The drawing under review shows one solid part. Ordinate dimensions are in mm from its lowest x, y, z. A direction names the side the tool comes from. Coordinates: 2 decimals unless noted, no trailing zeros. Loops run counter-clockwise (first coordinate to the right, second up) from the corner with the lowest first, then second, coordinate; pieces in that order, holes last. Notation, with made-up numbers: (24, -38) - (28, -38) arc R23 ccw to (28, -10) - close; hole circle Ø10 at (55, 48). An arc over 180 degrees is marked (long way). Use one line per item in the form item = value. Start each with the question number.
1. Machinability: for the marked faces 1 and 2, which of the approach directions +Z, -Z, +X, -X, +Y, -Y give a long, thin tool a straight path to every point of the face, cutting with its end or side? Answer none if there is none.
2. Add section C-C on z = 15. Give the boundary of the cut face in (x, y).
3. Add section B-B on x = 21. Give the boundary of the cut face in (y, z), and give its area (3 significant figures).
4. Add section A-A on y = 29.5. Give the boundary of the cut face in (x, z).
5. Add section D-D on z = 5.5. Give the boundary of the cut face in (x, y).
6. For pin 1 Ø3 at (x, z) = (21, 15) entering from +Y; pin 2 Ø1 at (x, z) = (31.5, 15.5) entering from +Y; pin 3 Ø15 at (y, z) = (29, 20) entering from +X, all flat-tipped, find the tip position at first contact; note any pin that passes through.
7. To check wall thickness, follow probe 1 along Z at (x, y) = (1.6, 29.5); probe 2 along X at (y, z) = (1.15, 15); probe 3 along Y at (x, z) = (24, 12.25). State the ranges of each line that lie inside material, in increasing order.
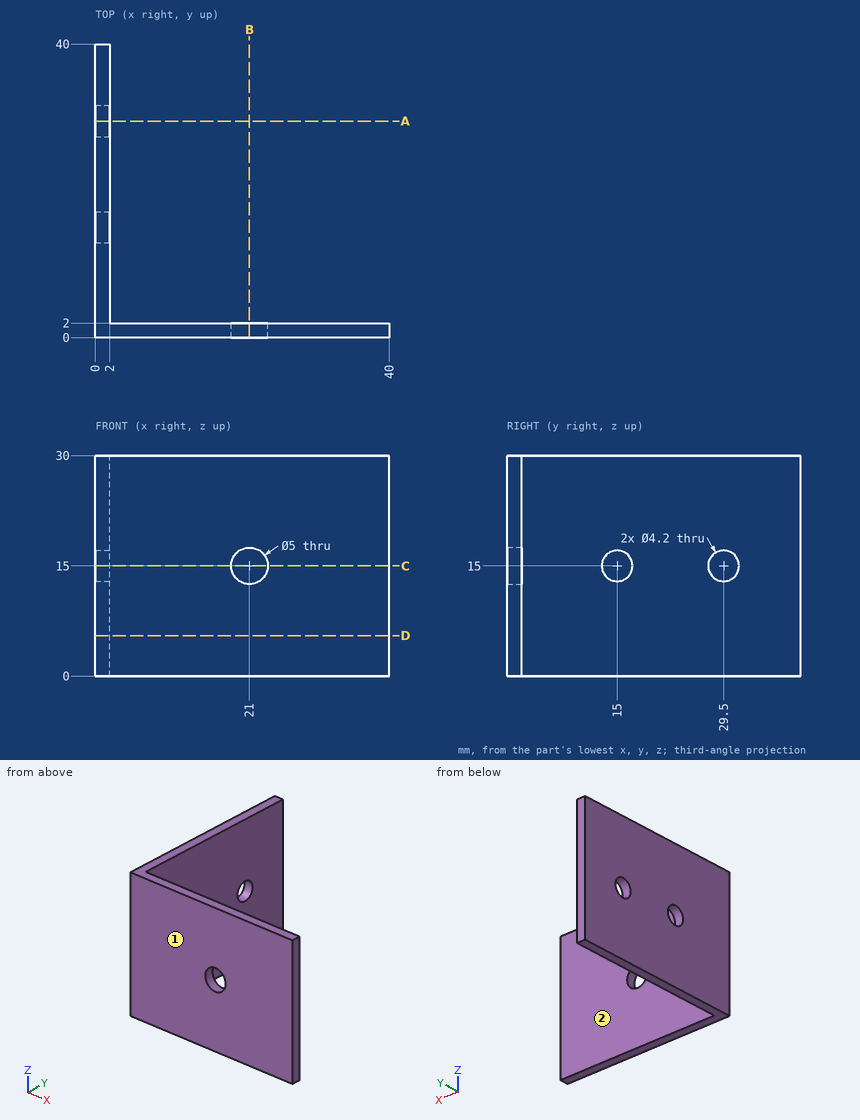
Conclusion:
q1.face_1 = +Z, -Z, +X, -X, -Y
q1.face_2 = +Z, -Z, +X, +Y
q2.outline = (0, 0) - (18.5, 0) - (18.5, 2) - (2, 2) - (2, 12.9) - (0, 12.9) - close; (0, 17.1) - (2, 17.1) - (2, 27.4) - (0, 27.4) - close; (0, 31.6) - (2, 31.6) - (2, 40) - (0, 40) - close; (23.5, 0) - (40, 0) - (40, 2) - (23.5, 2) - close
q3.outline = (0, 0) - (2, 0) - (2, 12.5) - (0, 12.5) - close; (0, 17.5) - (2, 17.5) - (2, 30) - (0, 30) - close
q3.area = 50.0 mm^2
q4.outline = (0, 0) - (2, 0) - (2, 12.9) - (0, 12.9) - close; (0, 17.1) - (2, 17.1) - (2, 30) - (0, 30) - close
q5.outline = (0, 0) - (40, 0) - (40, 2) - (2, 2) - (2, 40) - (0, 40) - close
q6.pin_1 = through
q6.pin_2 = 2
q6.pin_3 = 2
q7.probe_1 = 0 to 12.9, 17.1 to 30
q7.probe_2 = 0 to 18.5, 23.5 to 40
q7.probe_3 = 0 to 2
